For this review, use the dimensioned drawing (mm, ordinates from the lowest corner) and the shaded views. Round coordinates to 2 decimals unless told otherwise and drop trailing zeros. Loops run counter-clockwise (first coordinate to the right, second up) from the corner with the lowest first, then second, coordinate; pieces in that order, holes last. Notation, with made-up numbers: M 21.25,-20.75 L 25.25,-20.75 A31 cw 25.25,8.25 Z; hole C -20.5,-22.75 d7. An arc over 180 degrees is marked long. Answer as a JSON object with one key per item and string values. Group by question number.
Item 1: Consider section C-C (z = 1.05). Give the boundary of the cut face in (x, y) (3 decimals).
Item 2: To check wall thickness, follow line 1 (Y direction, x = 11.7, z = 0.1); line 2 (Y direction, x = 11.7, z = 0.95) (3 decimals); line 3 (Y direction, x = 13.75, z = 0.2). State the ranges of each line that lie inside material, in increasing order.
Item 3: The part is to be moulded in two halves that separate along X. For the marked faces 1, 2 and 3, say which applies: +X half, -X half, draft (parallel to the pull), parting line (faces both ways), or undercut.
Item 4: Insertion check: P1, Ø1.5, axis at x = 14, y = 9, coming from the +Z side; P2, Ø0.5, axis at y = 18, z = 0, coming from the -X side; P3, Ø0.5, axis at x = 3, z = 0.5, coming from the +Y side; P4, Ø0.5, axis at y = 4, z = 0, coming from the -X side. Each pin has a flat end and moves straight along its axis. Give the tip position at first contact, or say it passes through.
Item 5: Consider section B-B (y = 5.75). Give the boundary of the cut face in (x, z), and give its area (3 significant figures).
Item 6: Consider section A-A (x = 6.5). Give the boundary of the cut face in (y, z).
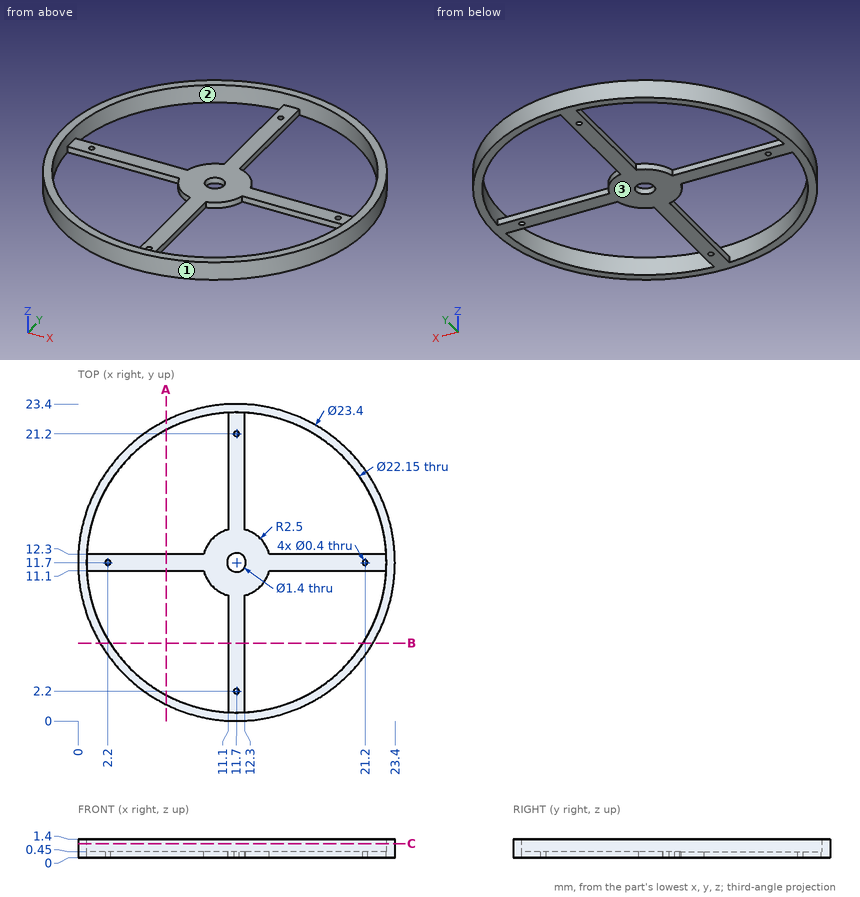
Geometry results:
{
 "1": {"outline": "C 11.7,11.7 d23.4; hole C 11.7,11.7 d22.15"},
 "2": {"line 1": "y = 0 to 2, 2.4 to 11, 12.4 to 21, 21.4 to 23.4", "line 2": "y = 0 to 0.625, 22.775 to 23.4", "line 3": "y = 0.18 to 0.82, 10.27 to 13.13, 22.58 to 23.22"},
 "3": {"face 1": "parting line", "face 2": "undercut", "face 3": "draft"},
 "4": {"P1": "passes through", "P2": "stops at x = 1.69", "P3": "stops at y = 19.79", "P4": "stops at x = 2.68"},
 "5": {"outline": "M 1.63,0 L 2.36,0 L 2.36,1.4 L 1.63,1.4 Z; M 11.1,0 L 12.3,0 L 12.3,0.45 L 11.1,0.45 Z; M 21.04,0 L 21.77,0 L 21.77,1.4 L 21.04,1.4 Z", "area": "2.59 mm^2"},
 "6": {"outline": "M 1.22,0 L 1.92,0 L 1.92,1.4 L 1.22,1.4 Z; M 11.1,0 L 12.3,0 L 12.3,0.45 L 11.1,0.45 Z; M 21.48,0 L 22.18,0 L 22.18,1.4 L 21.48,1.4 Z"}
}
